Source: CAD feature listing. Evaluate the final solid. Frame: model axes, mm. Round coordinates to 2 decimals unless told otherwise and drop trailing zeros. Loops run counter-clockwise (first coordinate to the right, second up) from the corner with the lowest first, then second, coordinate; pieces in that order, holes last. Notation, with made-up numbers: (4, -3.5) -> (14, -3.5) arc R20 cw to (14, 6.5) -> close; hole circle Ø9 at (-16, 8). An arc over 180 degrees is marked (long way). Put each result on its own line as item: value. Start each with the question number.
1. Cut plane D-D (z = -37). Return the cut outline in (x, y).
2. Contact query for flat-ended pins moving along their axis: pin 1 (2.5 mm diameter, centred on x = 0, z = 37, fed in from +Y) (1 decimal); pin 2 (1 mm diameter, centred on x = 25.5, y = 1, fed in from -Z). Output: stop coordinate, or through.
3. Material intervals for L1, parallel to X at y = 0.9, z = -18; L2, parallel to X at y = 2, z = -2; L3, parallel to X at y = 0.55, z = 17.5, sorted ascending.
4. Cut plane B-B (z = -18.5). Return the cut outline in (x, y), then the cut area to 3 significant figures.
5. Cut plane C-C (y = 2.45). State how many separate pieces and enclosed holes the cut face has, then the cut area to 3 significant figures.
6. Cut plane A-A (x = 0). Return the cut outline in (y, z), then the cut area to 3 significant figures.
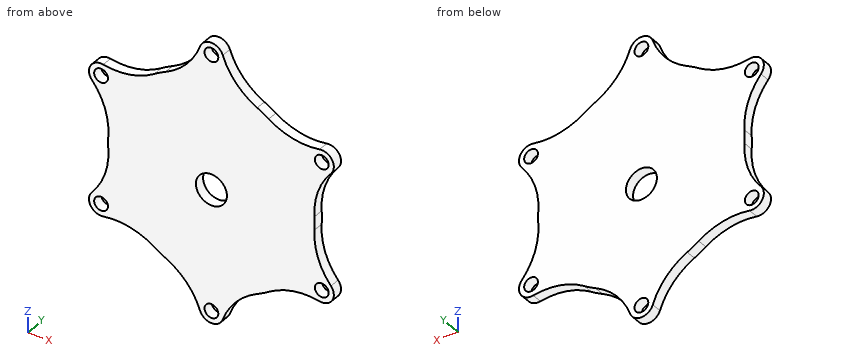
Autodesk Inventor part; units mm, degrees
ref_plane "XZ Plane" through (0, 0, 0) normal (0, 1, 0) x (-1, 0, 0)
sketch "Sketch1" plane through (0, 0, 0) normal (0, 1, 0) x (-1, 0, 0)
  circle A0 centre (0, 0) radius 30
  circle A1 centre (0, 0) radius 27.5
  circle A2 centre (0, -37) radius 3.5
  arc A3 (13.2962, -26.8926) -> (3.3005, -38.1648) centre (22.1604, -44.8209) ccw
  line L0 (0, -39.6745) -> (0, -15.9391) construction
  arc A4 (-3.3005, -38.1648) -> (-13.2962, -26.8926) centre (-22.1604, -44.8209) ccw
  line L1 (47.8103, 0) -> (-62.0389, 0) construction
  circle A5 centre (0, -37) radius 2
  circle A6 centre (32.0429, -18.5) radius 3.5
  circle A7 centre (32.0429, -18.5) radius 2
  arc A8 (31.4015, -21.9407) -> (16.6415, -24.9612) centre (27.7359, -41.6019) ccw
  arc A9 (29.9378, -1.9314) -> (34.7019, -16.2241) centre (49.8963, -3.219) ccw
  circle A10 centre (32.0429, 18.5) radius 3.5
  circle A11 centre (32.0429, 18.5) radius 2
  arc A12 (34.7019, 16.2241) -> (29.9378, 1.9314) centre (49.8963, 3.219) ccw
  arc A13 (16.6415, 24.9612) -> (31.4015, 21.9407) centre (27.7359, 41.6019) ccw
  circle A14 centre (0, 37) radius 3.5
  circle A15 centre (0, 37) radius 2
  arc A16 (3.3005, 38.1648) -> (13.2962, 26.8926) centre (22.1604, 44.8209) ccw
  arc A17 (-13.2962, 26.8926) -> (-3.3005, 38.1648) centre (-22.1604, 44.8209) ccw
  circle A18 centre (-32.0429, 18.5) radius 3.5
  circle A19 centre (-32.0429, 18.5) radius 2
  arc A20 (-31.4015, 21.9407) -> (-16.6415, 24.9612) centre (-27.7359, 41.6019) ccw
  arc A21 (-29.9378, 1.9314) -> (-34.7019, 16.2241) centre (-49.8963, 3.219) ccw
  circle A22 centre (-32.0429, -18.5) radius 3.5
  circle A23 centre (-32.0429, -18.5) radius 2
  arc A24 (-34.7019, -16.2241) -> (-29.9378, -1.9314) centre (-49.8963, -3.219) ccw
  arc A25 (-16.6415, -24.9612) -> (-31.4015, -21.9407) centre (-27.7359, -41.6019) ccw
  point P0 (29.9378, 1.9314)
  point P1 (34.7019, 16.2241)
  point P2 (16.6415, 24.9612)
  point P3 (13.2962, 26.8926)
  point P4 (3.3005, 38.1648)
  point P5 (-13.2962, 26.8926)
  point P6 (-29.9378, 1.9314)
  point P7 (-29.9378, -1.9314)
  point P8 (-16.6415, -24.9612)
  point P9 (-13.2962, -26.8926)
  point P10 (-3.3005, -38.1648)
  point P11 (16.6415, -24.9612)
  point P12 (31.4015, -21.9407)
  point P13 (29.9378, -1.9314)
  dimension "d16" = 60
  dimension "d18" = 7
  dimension "d17" = 55
  dimension "d19" = 37
  dimension "d21" = 20
  dimension "d22" = 4
  dimension "d25" = 360
extrude "Extrusion5" add sketch "Sketch1" along normal blind 3
extrude "Extrusion6" add sketch "Sketch1" along normal blind 3 contours A1
sketch "Sketch10" plane through (0, 3, 0) normal (0, 1, 0) x (1, 0, 0)
  circle A0 centre (0, 2) radius 4.5
  circle A1 centre (0, 2) radius 22.5
  point P0 (0, 0)
  dimension "d58" = 9
  dimension "d59" = 45
  dimension "d60" = 2
extrude "Extrusion12" cut sketch "Sketch10" against normal blind 20.25 contours A0
properties part number "carcaza motor"
Solution:
1. outline: (-3.75, 0) -> (-2, 0) -> (-2, 3) -> (-3.75, 3) -> close; (2, 0) -> (3.75, 0) -> (3.75, 3) -> (2, 3) -> close
2. pin 1: passes through
2. pin 2: stops at z = -21.79
3. L1: x = -35.51 to -33.98, -30.11 to 30.11, 33.98 to 35.51
3. L2: x = -29.93 to -4.5, 4.5 to 29.93
3. L3: x = -35.4 to -33.77, -30.31 to 30.31, 33.77 to 35.4
4. outline: (-35.54, 0) -> (-34.04, 0) -> (-34.04, 3) -> (-35.54, 3) -> close; (-30.04, 0) -> (30.04, 0) -> (30.04, 3) -> (-30.04, 3) -> close; (34.04, 0) -> (35.54, 0) -> (35.54, 3) -> (34.04, 3) -> close
4. area: 189 mm^2
5. separate pieces: 1
5. enclosed holes: 7
5. area: 3,370 mm^2
6. outline: (0, -40.5) -> (3, -40.5) -> (3, -39) -> (0, -39) -> close; (0, -35) -> (3, -35) -> (3, -6.5) -> (0, -6.5) -> close; (0, 2.5) -> (3, 2.5) -> (3, 35) -> (0, 35) -> close; (0, 39) -> (3, 39) -> (3, 40.5) -> (0, 40.5) -> close
6. area: 192 mm^2
